from build123d import *

# Parameters (mm, degrees)
SKETCH1_W           = 95.25
SKETCH1_H           = 127
BOSS_EXTRUDE1_DEPTH = 6.35
BOSS_EXTRUDE3_DEPTH = 6.35
SKETCH5_R           = 4.826
SKETCH5_R_2         = 5.039999953
SKETCH5_R_3         = 1.5
CUT_EXTRUDE1_DEPTH  = 7.35
CUT_EXTRUDE2_DEPTH  = 7.35
FILLET9_R           = 5
FILLET10_R          = 7.62
SKETCH7_R           = 2.2812375
CUT_EXTRUDE3_DEPTH  = 7.35
SKETCH8_R           = 1.5875
CUT_EXTRUDE4_DEPTH  = 7.35
SKETCH9_R           = 1.830008083
CUT_EXTRUDE5_DEPTH  = 7.35


with BuildPart() as part:
    # Sketch1 → Boss-Extrude1 (new body)
    with BuildSketch(Plane(origin=(0, 0, 0), x_dir=(1, 0, 0), z_dir=(0, 1, 0))):
        Rectangle(SKETCH1_W, SKETCH1_H)
    extrude(amount=BOSS_EXTRUDE1_DEPTH)

    # Sketch4 → Boss-Extrude3 (add)
    with BuildSketch(Plane(origin=(0, 6.35, 0), x_dir=(1, 0, 0), z_dir=(0, 1, 0))):
        with BuildLine():
            Line((-47.625, 63.5), (-171.916018217, 24.219268021))
            ThreePointArc((-171.916018217, 24.219268021), (-189.6618, 0), (-171.916018217, -24.219268021))
            Line((-171.916018217, -24.219268021), (-47.625, -63.5))
            Line((-47.625, -63.5), (-47.625, 63.5))
        make_face()
    extrude(amount=-BOSS_EXTRUDE3_DEPTH)

    # Sketch5 → Cut-Extrude1 (cut, through all)
    with BuildSketch(Plane(origin=(0, 6.35, 0), x_dir=(1, 0, 0), z_dir=(0, 1, 0))):
        with Locations((-164.2618, 0)):
            Circle(SKETCH5_R)
        with Locations((-48.9458, 0)):
            Circle(SKETCH5_R_2)
        with Locations((-40.106965235, 8.838834765)):
            Circle(SKETCH5_R_3)
        with Locations((-57.784634765, -8.838834765)):
            Circle(SKETCH5_R_3)
        with Locations((-55.663314421, 6.717514421)):
            Circle(SKETCH5_R_3)
        with Locations((-42.228285579, -6.717514421)):
            Circle(SKETCH5_R_3)
    extrude(amount=-CUT_EXTRUDE1_DEPTH, mode=Mode.SUBTRACT)

    # Sketch6 → Cut-Extrude2 (cut, through all)
    with BuildSketch(Plane(origin=(0, 6.35, 0), x_dir=(1, 0, 0), z_dir=(0, 1, 0))):
        Polygon((-63.5, 45.163743355), (-157.9118, 6.35), (-63.5, 6.35), align=None)
        Polygon((-63.5, -6.35), (-63.5, -45.163743355), (-157.9118, -6.35), align=None)
    extrude(amount=-CUT_EXTRUDE2_DEPTH, mode=Mode.SUBTRACT)

    # Fillet9
    fillet9_edges = [part.edges().sort_by_distance(p)[0] for p in [
        (-63.5, 3.175, -45.163743355),
        (-63.5, 3.175, -6.35),
        (-157.9118, 3.175, -6.35),
        (-157.9118, 3.175, 6.35),
        (-63.5, 3.175, 6.35),
        (-63.5, 3.175, 45.163743355),
    ]]
    fillet(fillet9_edges, radius=FILLET9_R)

    # Fillet10
    fillet10_edges = [part.edges().sort_by_distance(p)[0] for p in [
        (47.625, 3.175, 63.5),
        (47.625, 3.175, -63.5),
    ]]
    fillet(fillet10_edges, radius=FILLET10_R)

    # Sketch7 → Cut-Extrude3 (cut, through all)
    with BuildSketch(Plane(origin=(0, 6.35, 0), x_dir=(1, 0, 0), z_dir=(0, 1, 0))):
        with Locations((-43.777254611, -53.125383493)):
            Circle(SKETCH7_R)
        with Locations((-43.777254611, 53.125383493)):
            Circle(SKETCH7_R)
        with Locations((40.602254611, 53.125383493)):
            Circle(SKETCH7_R)
        with Locations((40.602254611, -53.125383493)):
            Circle(SKETCH7_R)
    extrude(amount=-CUT_EXTRUDE3_DEPTH, mode=Mode.SUBTRACT)

    # Sketch8 → Cut-Extrude4 (cut, through all)
    with BuildSketch(Plane(origin=(0, 6.35, 0), x_dir=(1, 0, 0), z_dir=(0, 1, 0))):
        with Locations((-13.209796215, -27.25)):
            Circle(SKETCH8_R)
        with Locations((8.564628211, -27.25)):
            Circle(SKETCH8_R)
        with Locations((8.564628211, -46.3)):
            Circle(SKETCH8_R)
        with Locations((-13.209796215, -46.3)):
            Circle(SKETCH8_R)
        with Locations((8.717854945, 46.8)):
            Circle(SKETCH8_R)
        with Locations((-13.056569481, 27.75)):
            Circle(SKETCH8_R)
        with Locations((-13.056569481, 46.8)):
            Circle(SKETCH8_R)
        with Locations((8.717854945, 27.75)):
            Circle(SKETCH8_R)
    extrude(amount=-CUT_EXTRUDE4_DEPTH, mode=Mode.SUBTRACT)

    # Sketch9 → Cut-Extrude5 (cut, through all)
    with BuildSketch(Plane(origin=(0, 6.35, 0), x_dir=(1, 0, 0), z_dir=(0, 1, 0))):
        with Locations((13.499388849, -20.49783886)):
            Circle(SKETCH9_R)
        with Locations((13.49951585, 20.502576943)):
            Circle(SKETCH9_R)
    extrude(amount=-CUT_EXTRUDE5_DEPTH, mode=Mode.SUBTRACT)


solid = part.part
The listing builds one solid part. Answer for the finished solid, in the listing's coordinates (mm). A direction names the side the tool comes from. Coordinates: 2 decimals unless noted, no trailing zeros. Write each loop counter-clockwise with the first axis right and the second up, starting at its lowest first coordinate (ties: lowest second). Pieces come first, ordered by that corner, then holes. Notation, with made-up numbers: M -13,-27 L 34,-27 A23 cw 34,3 Z; hole C -20.75,62.5 d4. An arc over 180 degrees is marked long. Write each question's results on one line, items separated by ' | '.
Item 1: For a pull along X with two mould halves and no side action, classify faces 3 (the face through (-4, 3, 63.5)), 4 (the face through (-44.139, 3.219, -1.514)), 5 (the face through (-110.641, 3.219, 43.585)), 6 (the face through (45.33, 3.22, -61.33)) as released by +X, released by -X, zero draft, split by the parting line, or undercut.
Answer below:
face 3: zero draft | face 4: undercut | face 5: released by -X | face 6: released by +X
Item 2: The part is cut by section A-A on z = 0. Determine the outline of the cut face in (x, y) (3 decimals), and give its area (3 significant figures).
Answer below:
outline: M -189.662,0 L -169.088,0 L -169.088,6.35 L -189.662,6.35 Z; M -159.436,0 L -53.986,0 L -53.986,6.35 L -159.436,6.35 Z; M -43.906,0 L 47.625,0 L 47.625,6.35 L -43.906,6.35 Z | area: 1,380 mm2
Item 3: Which of the six approach directions +Z, -Z, +X, -X, +Y, -Y give full straight-line access (tool end or side, diameter ignored) to faces 1 (the face through (45.45, 3.22, 61.21)), 2 (the face through (-101, 3, -6.35))?
Answer below:
face 1: +Z, +X, +Y, -Y | face 2: +Y, -Y
Item 4: The part is cut by section B-B on x = -113.5. Determine the outline of the cut face in (y, z).
Answer below:
outline: M 0,-42.68 L 6.35,-42.68 L 6.35,-24.61 L 0,-24.61 Z; M 0,-6.35 L 6.35,-6.35 L 6.35,6.35 L 0,6.35 Z; M 0,24.61 L 6.35,24.61 L 6.35,42.68 L 0,42.68 Z
Item 5: Given P1, Ø3.5, axis at x = -43.78, z = 53.13, coming from the -Y side; P2, Ø3.5, axis at x = -13.21, z = 27.25, coming from the +Y side; P3, Ø1.9, axis at x = -95, y = 3, coming from the +Z side, each flat-ended and moving along its own axis, determine where each tip first touches the part or whether it passes through.
Answer below:
P1: through | P2: y = 6.35 | P3: z = 48.83
Item 6: The part is cut by section C-C on y = 1. State how many separate pieces and enclosed holes the cut face has, and give its area (3 significant figures).
Answer below:
separate pieces: 1 | enclosed holes: 22 | area: 19,800 mm2
Item 7: Consider probe 1 along Z at (x, y) = (-132, 3.5); probe 2 along Z at (x, y) = (-118, 3.5); probe 3 along X at (y, z) = (0.5, 9) (3 decimals). Determine where each line is inside the solid, lowest interval first. Write a range as [from, to].
Answer below:
probe 1: [-36.83, -17], [-6.35, 6.35], [17, 36.83] | probe 2: [-41.26, -22.76], [-6.35, 6.35], [22.76, 41.26] | probe 3: [-188.014, -137.013], [-64.087, -59.276], [-56.293, 47.625]
